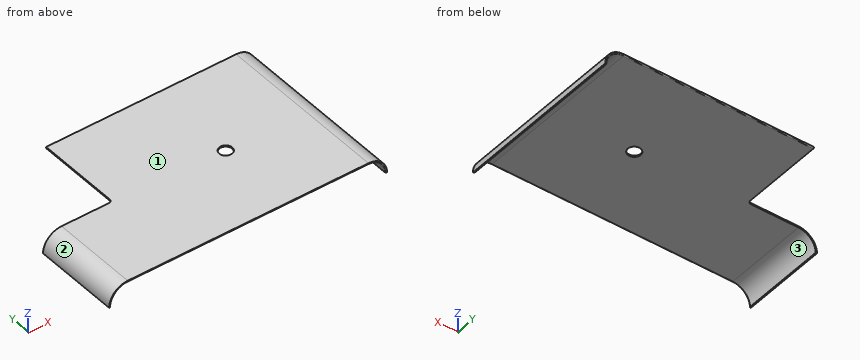
```python
from build123d import *

# Parameters (mm, degrees)
F1_DEPTH = 254
F3_DEPTH = 27.401
F4_W     = 101.6
F4_H     = 38.1
F5_DEPTH = 42.418
F6_R     = 1.27
F7_R     = 9.525
F8_DEPTH = 27.401


with BuildPart() as f1:
    # F0 (on Front) → F1 (new body)
    with BuildSketch(Plane.XZ):
        with BuildLine():
            ThreePointArc((-25.4, -25.4), (-17.960512, -7.439488), (0, 0))
            Line((0, 0), (355.6, 0))
            ThreePointArc((355.6, 0), (373.560512, -7.439488), (381, -25.4))
            Line((381, -25.4), (383, -25.4))
            ThreePointArc((383, -25.4), (374.974726, -6.025274), (355.6, 2))
            Line((355.6, 2), (0, 2))
            ThreePointArc((0, 2), (-19.374726, -6.025274), (-27.4, -25.4))
            Line((-27.4, -25.4), (-25.4, -25.4))
        make_face()
    extrude(amount=F1_DEPTH)

    # F2 (on face) → F3 (cut, through all)
    with BuildSketch(Plane.XY.offset(2)):
        with BuildLine():
            Line((74.93, 0), (50.8, 0))
            Line((50.8, 0), (-52.07, 0))
            Line((-52.07, 0), (-52.07, -101.6))
            Line((-52.07, -101.6), (-52.07, -127))
            Line((-52.07, -127), (0, -127))
            Line((0, -127), (69.85, -127))
            ThreePointArc((69.85, -127), (73.442102, -125.512102), (74.93, -121.92))
            Line((74.93, -121.92), (74.93, -25.4))
            Line((74.93, -25.4), (74.93, 0))
        make_face()
    extrude(amount=-F3_DEPTH, mode=Mode.SUBTRACT)

    # F4 (on Right) → F5 (cut)
    with BuildSketch(Plane.YZ):
        with Locations((-50.8, -19.05)):
            Rectangle(F4_W, F4_H)
    extrude(amount=-F5_DEPTH, mode=Mode.SUBTRACT)

    # F6
    f6_edges = [f1.edges().sort_by_distance(p)[0] for p in [
        (177.8, -254, 0),
        (215.265, 0, 0),
    ]]
    fillet(f6_edges, radius=F6_R)

    # F7 (on face) → F8 (cut, through all)
    with BuildSketch(Plane.XY.offset(2)):
        with Locations((237.59414, -133.37032)):
            Circle(F7_R)
    extrude(amount=-F8_DEPTH, mode=Mode.SUBTRACT)


solid = f1.part
```
Work out the finished part from the listing and answer in its coordinate system (mm). Face numbers are marked on the shaded views. Give positions to 0.01 mm unless a question says otherwise; leave off trailing zeros. Loops run counter-clockwise (first coordinate to the right, second up) from the corner with the lowest first, then second, coordinate; pieces in that order, holes last. Notation, with made-up numbers: M 39.5,42.5 L 53.5,42.5 A34 cw 53.5,77.5 Z; hole C -31.5,89.5 d8. An arc over 180 degrees is marked long. One line per item, written item: value. Start each with the question number.
1. Determine the mould class of the marked faces 1, 2 and 3 for opening direction X: released by +X, released by -X, zero draft, split by the parting line, or undercut.
2. Each of these flat-tipped pins is pushed along its axis until it touches: P1, Ø6, axis at x = 133.5, y = -97.5, coming from the -Z side; P2, Ø1.5, axis at y = -212, z = -12, coming from the -X side; P3, Ø8, axis at y = -103.5, z = -6, coming from the +X side. Where does it stop, or does it pass through?
3. Find the intervals of material crossed by probe 1 along Z at (x, y) = (318, -161); probe 2 along X at (y, z) = (-146.5, -15.25); probe 3 along X at (y, z) = (-205.5, -4), in increasing order.
4. Find section B-B (x = 30). Give the vertices of the cut face in (y, z), and give its area (3 significant figures).
5. Find section A-A (y = -182). Give the vertices of the cut face in (x, z).
6. Find section D-D (x = 264). Give the vertices of the cut face in (y, z), and give its area (3 significant figures).
7. Find section C-C (y = -93). Give the vertices of the cut face in (x, z).
Reported:
1. face 1: zero draft
1. face 2: released by -X
1. face 3: undercut
2. P1: stops at z = 0
2. P2: stops at x = -24.31
2. P3: stops at x = 378.26
3. probe 1: z = 0 to 2
3. probe 2: x = -25.45 to -23.28, 378.88 to 381.05
3. probe 3: x = -17.11 to -13.68, 369.28 to 372.71
4. outline: M -254,1.27 A1.27 ccw -252.73,0 L -127,0 L -127,2 L -254,2 Z
4. area: 254 mm²
5. outline: M -27.4,-25.4 L -25.4,-25.4 A25.4 cw 0,0 L 355.6,0 A25.4 cw 381,-25.4 L 383,-25.4 A27.4 ccw 355.6,2 L 0,2 A27.4 ccw Z
6. outline: M -254,1.27 A1.27 ccw -252.73,0 L -1.27,0 A1.27 ccw 0,1.27 L 0,2 L -254,2 Z
6. area: 507 mm²
7. outline: M 74.93,0 L 355.6,0 A25.4 cw 381,-25.4 L 383,-25.4 A27.4 ccw 355.6,2 L 74.93,2 Z
